The model under review builds one solid part; all positions refer to its coordinate system, in mm. A direction names the side the tool comes from. Round coordinates to 2 decimals unless told otherwise and drop trailing zeros. Write each loop counter-clockwise with the first axis right and the second up, starting at its lowest first coordinate (ties: lowest second). Pieces come first, ordered by that corner, then holes. Notation, with made-up numbers: (4, -6.75) - (46, -6.75) arc R26 cw to (46, 15.25) - close; hole circle Ø11 at (-8.5, 9). An arc over 180 degrees is marked (long way). One line per question, with ' | ' between items. Start each with the question number.
```python
from build123d import *

# Parameters (mm, degrees)
CROQUIS1_W              = 25
CROQUIS1_H              = 30
CROQUIS1_R              = 1.55
SALIENTE_EXTRUIR1_DEPTH = 23
CORTAR_EXTRUIR1_REACH   = 47.321
CROQUIS2_W              = 9
CROQUIS2_H              = 16.632666969
CORTAR_EXTRUIR2_REACH   = 47.321
CROQUIS3_R              = 2.575
CORTAR_EXTRUIR3_DEPTH   = 2.5
CROQUIS5_R              = 4.25
CORTAR_EXTRUIR4_DEPTH   = 4.5
CORTAR_EXTRUIR5_DEPTH   = 4.5
CORTAR_EXTRUIR6_REACH   = 47.321
REDONDEO3_R             = 1
CROQUIS8_R              = 2.575
CROQUIS8_R_2            = 2.05
SALIENTE_EXTRUIR2_DEPTH = 2.9
CORTAR_EXTRUIR7_DEPTH   = 1.5
CORTAR_EXTRUIR8_START   = -16.632667
CROQUIS10_W             = 1
CROQUIS10_H             = 30
CORTAR_EXTRUIR8_DEPTH   = 16.632667
REDONDEO4_R             = 5
REDONDEO5_R             = 2


with BuildPart() as part:
    # Croquis1 → Saliente-Extruir1 (new body)
    with BuildSketch(Plane(origin=(0, 0, 0), x_dir=(1, 0, 0), z_dir=(0, 1, 0))):
        with Locations((12.5, 15)):
            Rectangle(CROQUIS1_W, CROQUIS1_H)
        with Locations(Location((12.5, 25, 0), (0, 0, 270))):
            Circle(CROQUIS1_R, mode=Mode.SUBTRACT)
        with Locations(Location((12.5, 5, 0), (0, 0, 270))):
            Circle(CROQUIS1_R, mode=Mode.SUBTRACT)
    extrude(amount=SALIENTE_EXTRUIR1_DEPTH)

    # Cortar-Extruir1: up to this face of the body (flat: up to its plane)
    cortar_extruir1_end = Plane(part.part.faces().sort_by_distance((12.5, 11.5, 0))[0])
    # Croquis2 → Cortar-Extruir1 (cut, up to the picked face)
    with BuildSketch(Plane(origin=(0, 0, -30), x_dir=(-1, 0, 0), z_dir=(0, 0, -1)), mode=Mode.PRIVATE) as cortar_extruir1_sk1:
        with Locations((-12.5, 14.683666516)):
            Rectangle(CROQUIS2_W, CROQUIS2_H)
    cortar_extruir1_tool1 = split(extrude(cortar_extruir1_sk1.sketch, amount=-CORTAR_EXTRUIR1_REACH, mode=Mode.PRIVATE), bisect_by=cortar_extruir1_end, keep=Keep.BOTH, mode=Mode.PRIVATE)
    add(cortar_extruir1_tool1.solids().sort_by(Axis((12.5, 14.683667, -30), (0, 0, 1)))[0], mode=Mode.SUBTRACT)

    # Cortar-Extruir2: up to this face of the body (flat: up to its plane)
    cortar_extruir2_end = Plane(part.part.faces().sort_by_distance((25, 11.5, -15))[0])
    # Croquis3 → Cortar-Extruir2 (cut, up to the picked face)
    with BuildSketch(Plane.ZY, mode=Mode.PRIVATE) as cortar_extruir2_sk1:
        with Locations((-15, 16.5)):
            Circle(CROQUIS3_R)
    cortar_extruir2_tool1 = split(extrude(cortar_extruir2_sk1.sketch, amount=-CORTAR_EXTRUIR2_REACH, mode=Mode.PRIVATE), bisect_by=cortar_extruir2_end, keep=Keep.BOTH, mode=Mode.PRIVATE)
    add(cortar_extruir2_tool1.solids().sort_by(Axis((0, 16.5, -15), (1, 0, 0)))[0], mode=Mode.SUBTRACT)

    # Croquis4 → Cortar-Extruir3 (cut)
    with BuildSketch(Plane.ZY):
        Polygon((-14.95180736, 20.541164535), (-18.475654829, 18.562318318), (-18.523847469, 14.521153783), (-15.04819264, 12.458835465), (-11.524345171, 14.437681682), (-11.476152531, 18.478846217), align=None)
    extrude(amount=-CORTAR_EXTRUIR3_DEPTH, mode=Mode.SUBTRACT)

    # Croquis5 → Cortar-Extruir4 (cut)
    with BuildSketch(Plane(origin=(25, 0, 0), x_dir=(0, 0, -1), z_dir=(1, 0, 0))):
        with Locations((15, 16.5)):
            Circle(CROQUIS5_R)
    extrude(amount=-CORTAR_EXTRUIR4_DEPTH, mode=Mode.SUBTRACT)

    # Croquis6 → Cortar-Extruir5 (cut)
    with BuildSketch(Plane(origin=(0, 6.367333031, 0), x_dir=(1, 0, 0), z_dir=(0, 1, 0))):
        Polygon((15.848631561, 25), (14.174315781, 27.9), (10.825684219, 27.9), (9.151368439, 25), (10.825684219, 22.1), (14.174315781, 22.1), align=None)
        Polygon((15.848631561, 5), (14.174315781, 7.9), (10.825684219, 7.9), (9.151368439, 5), (10.825684219, 2.1), (14.174315781, 2.1), align=None)
    extrude(amount=-CORTAR_EXTRUIR5_DEPTH, mode=Mode.SUBTRACT)

    # Cortar-Extruir6: up to this face of the body (flat: up to its plane)
    cortar_extruir6_end = Plane(part.part.faces().sort_by_distance((25, 11.051957593, -15))[0])
    # Croquis7 → Cortar-Extruir6 (cut, up to the picked face)
    with BuildSketch(Plane.ZY, mode=Mode.PRIVATE) as cortar_extruir6_sk1:
        with BuildLine():
            Line((-22.745966692, 23), (-30, 23))
            Line((-30, 23), (-30, 8))
            ThreePointArc((-30, 8), (-27.536048339, 16.062460813), (-22.745966692, 23))
        make_face()
    cortar_extruir6_tool1 = split(extrude(cortar_extruir6_sk1.sketch, amount=-CORTAR_EXTRUIR6_REACH, mode=Mode.PRIVATE), bisect_by=cortar_extruir6_end, keep=Keep.BOTH, mode=Mode.PRIVATE)
    # Croquis7 → Cortar-Extruir6 (cut, up to the picked face)
    with BuildSketch(Plane.ZY, mode=Mode.PRIVATE) as cortar_extruir6_sk2:
        with BuildLine():
            Line((0, 23), (-7.254033308, 23))
            ThreePointArc((-7.254033308, 23), (-2.463951661, 16.062460813), (0, 8))
            Line((0, 8), (0, 23))
        make_face()
    cortar_extruir6_tool2 = split(extrude(cortar_extruir6_sk2.sketch, amount=-CORTAR_EXTRUIR6_REACH, mode=Mode.PRIVATE), bisect_by=cortar_extruir6_end, keep=Keep.BOTH, mode=Mode.PRIVATE)
    add(cortar_extruir6_tool1.solids().sort_by(Axis((0, 18.820242, -27.849866), (1, 0, 0)))[0], mode=Mode.SUBTRACT)
    add(cortar_extruir6_tool2.solids().sort_by(Axis((0, 18.820242, -2.150134), (1, 0, 0)))[0], mode=Mode.SUBTRACT)

    # Redondeo3
    redondeo3_edges = [part.edges().sort_by_distance(p)[0] for p in [
        (25, 4, -30),
        (0, 4, -30),
        (25, 4, 0),
        (0, 4, 0),
    ]]
    fillet(redondeo3_edges, radius=REDONDEO3_R)

    # Croquis8 → Saliente-Extruir2 (add)
    with BuildSketch(Plane.ZY.offset(-2.5)):
        with Locations((-15, 16.5)):
            Circle(CROQUIS8_R)
        with Locations((-15, 16.5)):
            Circle(CROQUIS8_R_2, mode=Mode.SUBTRACT)
    extrude(amount=-SALIENTE_EXTRUIR2_DEPTH)

    # Croquis9 → Cortar-Extruir7 (cut)
    with BuildSketch(Plane.ZY.offset(-2.5)):
        Polygon((-11.476152531, 18.478846217), (-14.95180736, 20.541164535), (-18.475654829, 18.562318318), (-18.523847469, 14.521153783), (-15.04819264, 12.458835465), (-11.524345171, 14.437681682), align=None)
    extrude(amount=-CORTAR_EXTRUIR7_DEPTH, mode=Mode.SUBTRACT)

    # Croquis10 → Cortar-Extruir8 (cut)
    with BuildSketch(Plane(origin=(0, 23, 0), x_dir=(1, 0, 0), z_dir=(0, 1, 0)).offset(CORTAR_EXTRUIR8_START)):
        with Locations((17.5, 15)):
            Rectangle(CROQUIS10_W, CROQUIS10_H)
        with Locations((7.5, 15)):
            Rectangle(CROQUIS10_W, CROQUIS10_H)
    extrude(amount=CORTAR_EXTRUIR8_DEPTH, mode=Mode.SUBTRACT)

    # Redondeo4
    redondeo4_edges = [part.edges().sort_by_distance(p)[0] for p in [
        (21.5, 23, -22.745966692),
        (21.5, 23, -7.254033308),
        (3.5, 23, -22.745966692),
        (3.5, 23, -7.254033308),
    ]]
    fillet(redondeo4_edges, radius=REDONDEO4_R)

    # Redondeo5
    # the kernel refuses this fillet: 2 mm, written as the material it adds along each edge
    with BuildSketch(Plane(origin=(7, 6.367333, 0), x_dir=(1, 0, 0), z_dir=(0, 0, -1))) as redondeo5_piece_1_section:
        with BuildLine():
            CenterArc((REDONDEO5_R, -REDONDEO5_R), REDONDEO5_R, 90, 90)
            Line((0, -REDONDEO5_R), (0, 0))
            Line((0, 0), (REDONDEO5_R, 0))
        make_face()
    redondeo5_piece_1 = extrude(amount=30, mode=Mode.PRIVATE)
    redondeo5_piece_1 = redondeo5_piece_1 & Plane(origin=(7.452804223, 4.086860333, -2.772720189), x_dir=(0, 0.14225955268543314, -0.9898293891725687), z_dir=(-1, 0, 0)) * Cylinder(27.507043243, 68, mode=Mode.PRIVATE)
    redondeo5_piece_1 = redondeo5_piece_1 & Plane(origin=(7.452804223, 4.086860333, -27.227279811), x_dir=(0, 0.6875744332215433, 0.7261139020705178), z_dir=(-1, 0, 0)) * Cylinder(27.507043243, 68, mode=Mode.PRIVATE)
    add(redondeo5_piece_1)
    with BuildSketch(Plane(origin=(18, 6.367333, 0), x_dir=(0, 1, 0), z_dir=(0, 0, -1))) as redondeo5_piece_2_section:
        with BuildLine():
            CenterArc((REDONDEO5_R, -REDONDEO5_R), REDONDEO5_R, 90, 90)
            Line((0, -REDONDEO5_R), (0, 0))
            Line((0, 0), (REDONDEO5_R, 0))
        make_face()
    redondeo5_piece_2 = extrude(amount=30, mode=Mode.PRIVATE)
    redondeo5_piece_2 = redondeo5_piece_2 & Plane(origin=(17.547195777, 4.086860333, -27.227279811), x_dir=(0, 0.6875744332215433, 0.7261139020705178), z_dir=(-1, 0, 0)) * Cylinder(27.507043243, 69, mode=Mode.PRIVATE)
    redondeo5_piece_2 = redondeo5_piece_2 & Plane(origin=(17.547195777, 4.086860333, -2.772720189), x_dir=(0, 0.14225955268543314, -0.9898293891725687), z_dir=(-1, 0, 0)) * Cylinder(27.507043243, 69, mode=Mode.PRIVATE)
    add(redondeo5_piece_2)


solid = part.part
```
1. Add section C-C, the plane z = -24. Write out the cut boundary in (x, y), then the cut area to 3 significant figures.
2. Clearance check with flat-ended pins moving along their axes: P1, Ø4, axis at x = 6, y = 11.5, coming from the +Z side; P2, Ø2, axis at x = 11, z = -22.5, coming from the +Y side; P3, Ø3, axis at y = 15.5, z = -13, coming from the +X side. State where each tip first meets the part, or that it passes through.
3. Wall thickness on line 1 along Z through (x, y) = (12.5, 1.3); line 2 along X through (y, z) = (1.15, -25); line 3 along X through (y, z) = (20, -7): over which ranges is each line inside the solid? List them lowest first. Write a range as [from, to].
4. The part is to be moulded in two halves that separate along X. For faces 6 (the face through (13, 4, 0)), 7 (the face through (12, 6.367, -15)), 8 (the face through (0.285, 4.901, -0.301)), say which applies: pulls with the +X half, pulls with the -X half, needs draft (parallel to the pull), parting line crosses it, or undercut.
5. Add section D-D, the plane y = 16.5. Write out the cut boundary in (x, z) (3 decimals).
6. Add section A-A, the plane y = 4. Write out the cut boundary in (x, z).
7. Machinability: for faces 1 (the face through (20.5, 13.7, -14.9)), 2 (the face through (21, 23, -15)), 3 (the face through (15, 4.15, -23.53)), 4 (the face through (7, 12, -15)), 5 (the face through (2, 19.5, -13.2)), which of the approach directions +Z, -Z, +X, -X, +Y, -Y give a long, thin tool a straight path to every point of the face, cutting with its end or side? Answer none if there is none.
8. Add section B-B, the plane x = 12.5. Write out the cut boundary in (y, z), then the cut area to 3 significant figures.
Geometry check:
1) outline: (0, 0) - (11.32, 0) - (11.32, 1.87) - (9.73, 1.87) - (9.73, 6.37) - (9, 6.37) arc R2 cw to (7, 8.37) - (7, 21.54) - (0, 21.54) - close; (13.68, 0) - (25, 0) - (25, 21.54) - (18, 21.54) - (18, 8.37) arc R2 cw to (16, 6.37) - (15.27, 6.37) - (15.27, 1.87) - (13.68, 1.87) - close | area: 344 mm2
2) P1: stops at z = -0.26 | P2: stops at y = 6.37 | P3: stops at x = 20.5
3) line 1: z = [-30, -26.55], [-23.45, -6.55], [-3.45, 0] | line 2: x = [0, 10.95], [14.05, 25] | line 3: x = [0, 7], [18, 25]
4) face 6: needs draft | face 7: undercut | face 8: pulls with the -X half
5) outline: (0, -27.32) - (7, -27.32) - (7, -17.575) - (5.4, -17.575) - (5.4, -17.05) - (4, -17.05) - (4, -18.5) - (0, -18.5) - close; (0, -11.5) - (4, -11.5) - (4, -12.95) - (5.4, -12.95) - (5.4, -12.425) - (7, -12.425) - (7, -2.68) - (0, -2.68) - close; (18, -27.32) - (25, -27.32) - (25, -19.25) - (20.5, -19.25) - (20.5, -17.575) - (18, -17.575) - close; (18, -12.425) - (20.5, -12.425) - (20.5, -10.75) - (25, -10.75) - (25, -2.68) - (18, -2.68) - close
6) outline: (0, -29) arc R1 ccw to (1, -30) - (24, -30) arc R1 ccw to (25, -29) - (25, -1) arc R1 ccw to (24, 0) - (1, 0) arc R1 ccw to (0, -1) - close; hole (9.15, -25) - (10.83, -27.9) - (14.17, -27.9) - (15.85, -25) - (14.17, -22.1) - (10.83, -22.1) - close; hole (9.15, -5) - (10.83, -7.9) - (14.17, -7.9) - (15.85, -5) - (14.17, -2.1) - (10.83, -2.1) - close
7) face 1: +X | face 2: +Z, -Z, +X, -X, +Y | face 3: +Y | face 4: +Z, -Z, +Y | face 5: -X
8) outline: (0, -30) - (6.37, -30) - (6.37, -27.9) - (1.87, -27.9) - (1.87, -26.55) - (0, -26.55) - close; (0, -23.45) - (1.87, -23.45) - (1.87, -22.1) - (6.37, -22.1) - (6.37, -7.9) - (1.87, -7.9) - (1.87, -6.55) - (0, -6.55) - close; (0, -3.45) - (1.87, -3.45) - (1.87, -2.1) - (6.37, -2.1) - (6.37, 0) - (0, 0) - close | area: 127 mm2
